The drawing under review shows one solid part. Ordinate dimensions are in mm from its lowest x, y, z. Round coordinates to 2 decimals unless told otherwise and drop trailing zeros. Order: outer loops, then holes, each group sorted by start corner. A loop starts at its lowest first (then second) coordinate and runs counter-clockwise, first axis right, second up. Notation, with made-up numbers: (64.5, 1) - (89.5, 1) arc R21 cw to (89.5, 13) - close; hole circle Ø5 at (33, -4.5). An arc over 180 degrees is marked (long way). Answer as a JSON object with one key per item and string values. Group by question number.
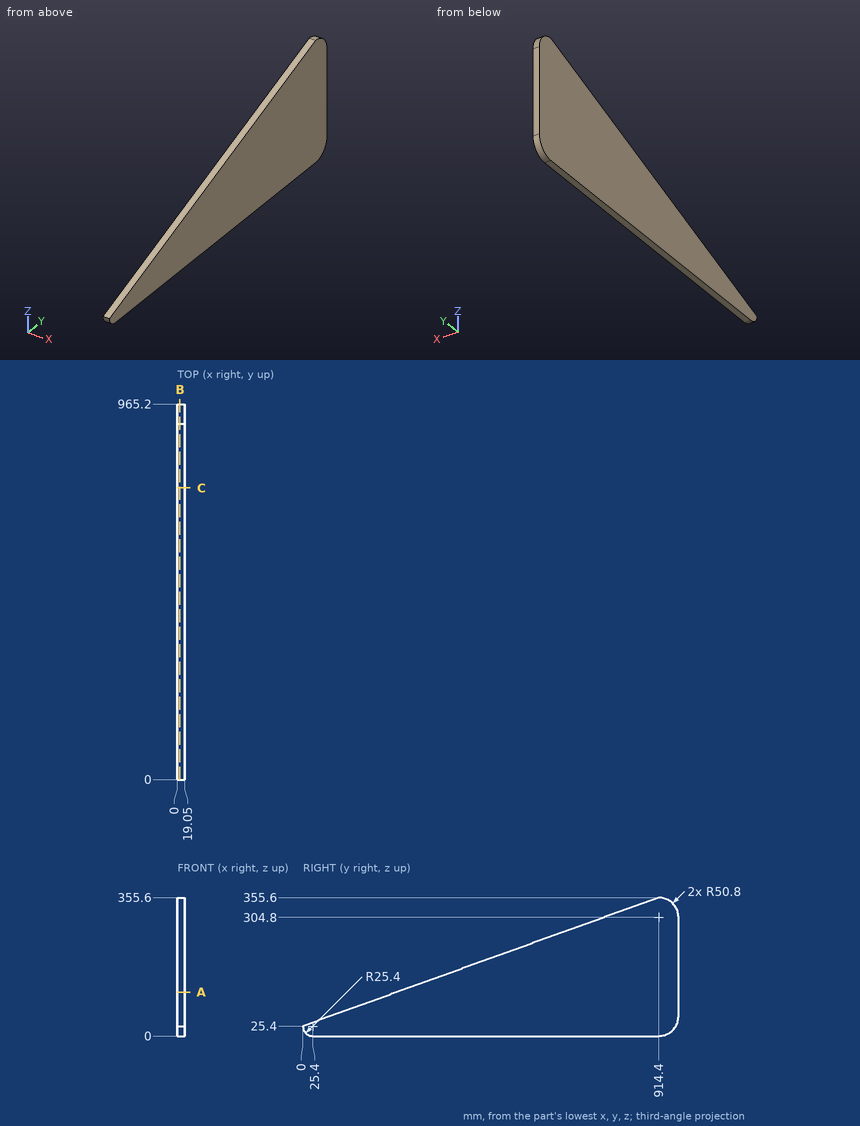
1. To check wall thickness, follow line 1 (Z direction, x = 15.25, y = 787); line 2 (Z direction, x = 3.75, y = 746.5). State the ranges of each line that lie inside material, in increasing order. Write a range as from..to.
2. Clearance check with a flat-ended pin moving along its axis: P1, Ø3, axis at x = 2, z = 315.5, coming from the +Y side. State where the tip first meets the part, or that it passes through.
3. Take a section at A-A, the plane z = 112.5. Give the boundary of the cut face in (x, y).
4. Take a section at C-C, the plane y = 749.5. Give the boundary of the cut face in (x, z), then the cut area to 3 significant figures.
5. Take a section at B-B, the plane x = 6. Give the boundary of the cut face in (y, z).
Response values:
{
 "1": {"line 1": "0..309.59", "line 2": "0..294.97"},
 "2": {"P1": "y = 964.36"},
 "3": {"outline": "(0, 241.2) - (19.05, 241.2) - (19.05, 965.2) - (0, 965.2) - close"},
 "4": {"outline": "(0, 0) - (19.05, 0) - (19.05, 296.05) - (0, 296.05) - close", "area": "5,640 mm2"},
 "5": {"outline": "(0, 25.4) arc R25.4 ccw to (25.4, 0) - (914.4, 0) arc R50.8 ccw to (965.2, 50.8) - (965.2, 304.8) arc R50.8 ccw to (914.4, 355.6) - close"}
}
